Can you work these out from the drawing? Everything is in mm from the part's minimum corner. Round coordinates to 2 decimals unless told otherwise and drop trailing zeros. Write each loop counter-clockwise with the first axis right and the second up, starting at its lowest first coordinate (ties: lowest second). Pieces come first, ordered by that corner, then holes. Notation, with made-up numbers: (66.5, 50) -> (124.5, 50) arc R18 ccw to (124.5, 67) -> close; hole circle Ø10 at (44.25, 53.5). An arc over 180 degrees is marked (long way). Answer as CSV lines item,"result". Start each with the question number.
Q1. Imagine slicing it at A-A on y = 2.5. Please give me the cut outline in (x, z).
Q2. If I drill on line 1 (Y direction, x = 0.3, z = 11), over which ranges is the centre line in solid material (lowest first)? Write a range as [from, to].
Q3. Imagine slicing it at C-C on x = 0.15. Please give me the cut outline in (y, z), and give its area (3 significant figures).
Q4. Imagine slicing it at B-B on z = 11. Please give me the cut outline in (x, y).
Q5. Imagine slicing it at D-D on y = 20.5. Please give me the cut outline in (x, z).
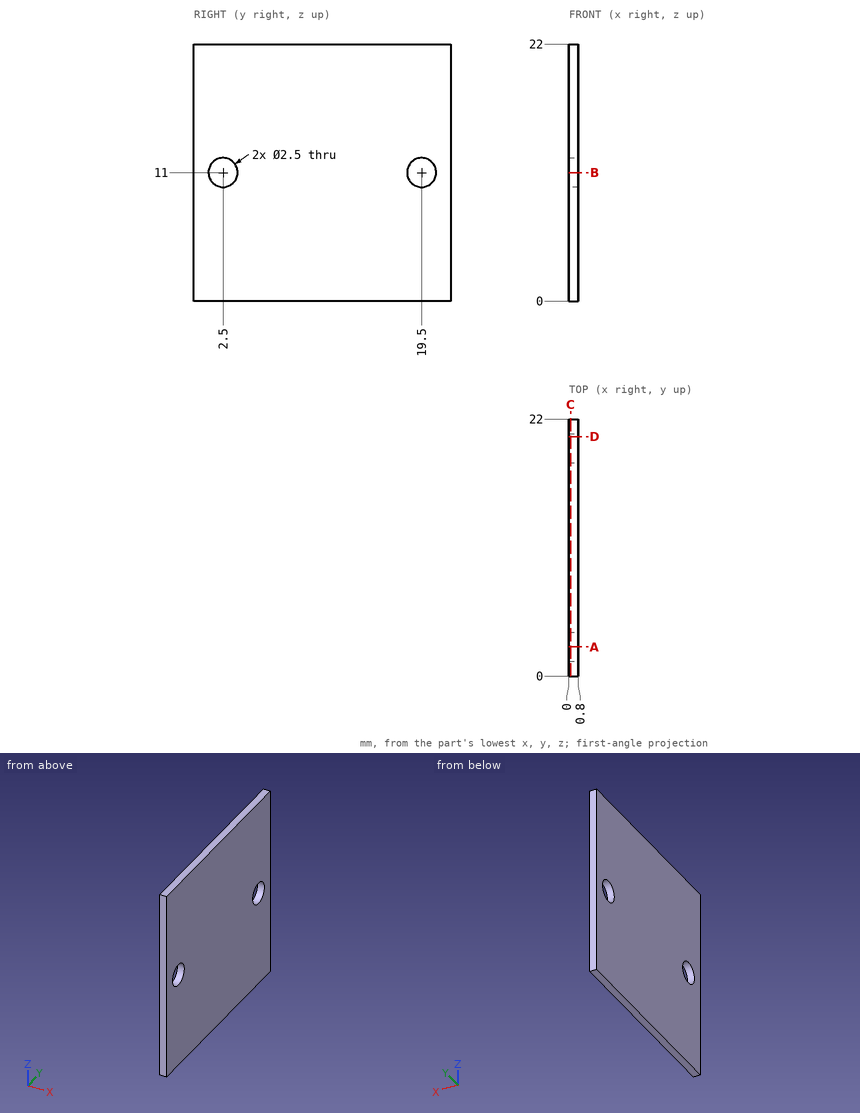
Checks:
1,outline,"(0, 0) -> (0.8, 0) -> (0.8, 9.75) -> (0, 9.75) -> close; (0, 12.25) -> (0.8, 12.25) -> (0.8, 22) -> (0, 22) -> close"
2,line 1,"[0, 1.25], [3.75, 18.25], [20.75, 22]"
3,outline,"(0, 0) -> (22, 0) -> (22, 22) -> (0, 22) -> close; hole circle Ø2.5 at (2.5, 11); hole circle Ø2.5 at (19.5, 11)"
3,area,"474 mm^2"
4,outline,"(0, 0) -> (0.8, 0) -> (0.8, 1.25) -> (0, 1.25) -> close; (0, 3.75) -> (0.8, 3.75) -> (0.8, 18.25) -> (0, 18.25) -> close; (0, 20.75) -> (0.8, 20.75) -> (0.8, 22) -> (0, 22) -> close"
5,outline,"(0, 0) -> (0.8, 0) -> (0.8, 10.25) -> (0, 10.25) -> close; (0, 11.75) -> (0.8, 11.75) -> (0.8, 22) -> (0, 22) -> close"
